from build123d import *

# Parameters (mm, degrees)
F1_W      = 70
F1_H      = 90
F2_DEPTH  = 33
F3_W      = 26
F3_H      = 15
F4_DEPTH  = 90.001
F5_DEPTH  = 24
F6_W      = 16
F6_H      = 25
F7_DEPTH  = 90.001
F8_R      = 20
F9_DEPTH  = 59.001
F10_W     = 28
F10_H     = 50
F11_DEPTH = 16


# Not quite as in the source:
# - a pattern or mirror of a feature is missing from the dataset's text; its kind, count and spacing are read off the source's solid


with BuildPart() as f2:
    # F1 (on Top) → F2 (new body)
    with BuildSketch(Plane.XY):
        Rectangle(F1_W, F1_H)
    extrude(amount=-F2_DEPTH)

    # F3 (on face) → F4 (cut, through all)
    with BuildSketch(Plane.XZ.offset(45)):
        with Locations((7, -25.5)):
            Rectangle(F3_W, F3_H)
    extrude(amount=-F4_DEPTH, mode=Mode.SUBTRACT)

    # F0 (on Right) → F5 (join, symmetric)
    with BuildSketch(Plane.YZ):
        Polygon((-25, 37), (-45, 0), (45, 0), (25, 37), align=None)
    extrude(amount=F5_DEPTH, both=True)

    # F6 (on face) → F7 (cut, through all)
    with BuildSketch(Plane.XZ.offset(45)):
        with Locations((0, 24.5)):
            Rectangle(F6_W, F6_H)
    extrude(amount=-F7_DEPTH, mode=Mode.SUBTRACT)

    # F8 (on face) → F9 (cut, through all)
    with BuildSketch(Plane.YZ.offset(24)):
        with Locations((0, 37)):
            Circle(F8_R)
    extrude(amount=-F9_DEPTH, mode=Mode.SUBTRACT)

    # F10 (on face) → F11 (cut)
    with BuildSketch(Plane.YZ.offset(35)):
        with Locations((0, 15.2474023402)):
            Rectangle(F10_W, F10_H)
    f11 = extrude(amount=-F11_DEPTH, mode=Mode.SUBTRACT)

    # F11_copies: F11 across plane
    add(f11.mirror(Plane(origin=(0, 0, 0), x_dir=(0, 0, -1), z_dir=(-1, 0, 0))), mode=Mode.SUBTRACT)


solid = f2.part
Verification items for the finished model (mm, model axes). A direction names the side the tool comes from. Coordinates: 2 decimals unless noted, no trailing zeros. Write each loop counter-clockwise with the first axis right and the second up, starting at its lowest first coordinate (ties: lowest second). Pieces come first, ordered by that corner, then holes. Notation, with made-up numbers: (12.25, 37) -> (29.25, 37) arc R18 ccw to (29.25, 72) -> close; hole circle Ø11 at (-10, 36.5). An arc over 180 degrees is marked (long way). One line per item, written item: value. Start each with the question number.
Q1. Access from +Z, -Z, +X, -X, +Y, -Y to the whole of each face (thin tool, end or side, straight path). Record for faces 1 (the flat face through (24, 26, 15)), 2 (the flat face through (19, 0, 3)), 3 (the flat face through (20, -1, -26)).
Q2. Go/stop test with flat-tipped pins: P1, Ø2, axis at y = 22.5, z = 7.5, coming from the -X side; P2, Ø13, axis at x = -30.5, y = 6, coming from the +Z side; P3, Ø8.5, axis at y = 1, z = 8.5, coming from the +X side. Record where each tip stops, or that it passes through.
Q3. Mould release check, pull along Y, two halves, no side actions. Record for faces 4 (the flat face through (-30, -29, 0)), 5 (the flat face through (0.336, -39.304, 10.537)), 6 (the flat face through (27, 0, -9.753)): pulls with the +Y half, pulls with the -Y half, needs draft (parallel to the pull), parting line crosses it, or undercut.
Q4. Cross-section at D-D on z = -7. Enter the section's corners in (x, y), and give its area (3 significant figures).
Q5. Cross-section at B-B on y = 33. Enter the section's corners in (x, z).
Q6. Cross-section at A-A on x = -12.5. Enter the section's corners in (y, z).
Q7. Thickness scan on L1, parallel to Y at x = -25, z = -3; L2, parallel to X at y = 28.5, z = -19; L3, parallel to X at y = -21, z = 18. Record the ranges inside material, lowest first. Write a range as from..to.
Q8. Cross-section at C-C on z = 32.5. Enter the section's corners in (x, y).
Checked values:
1. face 1: +Z, +X, +Y, -Y
1. face 2: +Z, +X
1. face 3: -Z, +Y, -Y
2. P1: stops at x = -24
2. P2: stops at z = -9.75
2. P3: stops at x = 19
3. face 4: needs draft
3. face 5: pulls with the -Y half
3. face 6: undercut
4. outline: (-35, -45) -> (35, -45) -> (35, -14) -> (19, -14) -> (19, 14) -> (35, 14) -> (35, 45) -> (-35, 45) -> (-35, 14) -> (-19, 14) -> (-19, -14) -> (-35, -14) -> close
4. area: 5,400 mm²
5. outline: (-35, -33) -> (-6, -33) -> (-6, -18) -> (20, -18) -> (20, -33) -> (35, -33) -> (35, 0) -> (24, 0) -> (24, 22.2) -> (8, 22.2) -> (8, 12) -> (-8, 12) -> (-8, 22.2) -> (-24, 22.2) -> (-24, 0) -> (-35, 0) -> close
6. outline: (-45, -33) -> (45, -33) -> (45, 0) -> (25, 37) -> (20, 37) arc R20 cw to (-20, 37) -> (-25, 37) -> (-45, 0) -> close
7. L1: y = -45..-14, 14..45
7. L2: x = -35..-6, 20..35
7. L3: x = -24..-8, 8..24
8. outline: (-24, -27.43) -> (-8, -27.43) -> (-8, -19.49) -> (-24, -19.49) -> close; (-24, 19.49) -> (-8, 19.49) -> (-8, 27.43) -> (-24, 27.43) -> close; (8, -27.43) -> (24, -27.43) -> (24, -19.49) -> (8, -19.49) -> close; (8, 19.49) -> (24, 19.49) -> (24, 27.43) -> (8, 27.43) -> close
